```python
from build123d import *

# Parameters (mm, degrees)
CYLINDER950_R          = 0.9
CYLINDER950_DEPTH      = 15
CYLINDER950_ROLL_ANGLE = 90
CYLINDER951_R          = 0.9
CYLINDER951_DEPTH      = 15
CYLINDER951_ROLL_ANGLE = 90
BOX558_W               = 5
BOX558_H               = 60
BOX558_DEPTH           = 17
BOX557_W               = 7
BOX557_H               = 15
BOX557_DEPTH           = 17
FILLET357_R            = 3


with BuildPart() as cylinder1101:
    # Cylinder950 → Cylinder950 (new body)
    with BuildSketch(Plane.XY):
        Circle(CYLINDER950_R)
    extrude(amount=CYLINDER950_DEPTH)


with BuildPart() as cylinder1101_1:
    # Cylinder950 roll: moved
    add(cylinder1101.part.rotate(Axis((0, 0, 0), (1, 0, 0)), CYLINDER950_ROLL_ANGLE))


with BuildPart() as cylinder1101_2:
    # Cylinder950 placement: moved
    add(cylinder1101_1.part.moved(Location((27, 85, -10.2))))


with BuildPart() as fusion596:
    # Cylinder951 → Cylinder951 (new body)
    with BuildSketch(Plane.XY):
        Circle(CYLINDER951_R)
    extrude(amount=CYLINDER951_DEPTH)


with BuildPart() as fusion596_1:
    # Cylinder951 roll: moved
    add(fusion596.part.rotate(Axis((0, 0, 0), (1, 0, 0)), CYLINDER951_ROLL_ANGLE))


with BuildPart() as fusion596_2:
    # Cylinder951 placement: moved
    add(fusion596_1.part.moved(Location((27, 85, 0))))

    # Fusion596: union Cylinder1101
    add(cylinder1101_2.part)


with BuildPart() as fusion596_3:
    # Fusion596 placement: moved
    add(fusion596_2.part.moved(Location((44.2, 9.5, -5.9))))


with BuildPart() as cube749:
    # Box558 → Box558 (new body)
    with BuildSketch(Plane(origin=(74.5, 55, -19.5), x_dir=(1, 0, 0), z_dir=(0, 0, 1))):
        with Locations((2.5, 30)):
            Rectangle(BOX558_W, BOX558_H)
    extrude(amount=BOX558_DEPTH)


with BuildPart() as steering_servo_rear_mount:
    # Box557 → Box557 (new body)
    with BuildSketch(Plane(origin=(67.5, 79.5, -19.5), x_dir=(1, 0, 0), z_dir=(0, 0, 1))):
        with Locations((3.5, 7.5)):
            Rectangle(BOX557_W, BOX557_H)
    extrude(amount=BOX557_DEPTH)

    # Fusion597: union Cube749
    add(cube749.part)

    # Cut695: cut Fusion596
    add(fusion596_3.part, mode=Mode.SUBTRACT)

    # Fillet357
    fillet357_edges = [steering_servo_rear_mount.edges().sort_by_distance(p)[0] for p in [
        (77, 55, -2.5),
        (77, 115, -2.5),
        (77, 115, -19.5),
        (77, 55, -19.5),
    ]]
    fillet(fillet357_edges, radius=FILLET357_R)


with BuildPart() as steering_servo_rear_mount_1:
    # Fillet357 placement: moved
    add(steering_servo_rear_mount.part.moved(Location((1, 0, 0))))


solid = steering_servo_rear_mount_1.part
```
CAD build for the part. Positions are in the model's coordinates, mm. A direction names the side the tool comes from. Coordinates: 2 decimals unless noted, no trailing zeros. Order: outer loops, then holes, each group sorted by start corner. A loop starts at its lowest first (then second) coordinate and runs counter-clockwise, first axis right, second up. Notation, with made-up numbers: M 10.25,46.5 L 19.25,46.5 A14 cw 19.25,69.5 Z; hole C 31,52.25 d7. An arc over 180 degrees is marked long. Answer as CSV lines item,"result".
1) Mould opens along Z. For faces 1 (the flat face through (77, 85, -2.5)), 2 (the flat face through (80.5, 85, -11)), 3 (the cylindrical face through (71.3, 87.1, -5.9)), 4 (the cylindrical face through (71.3, 87.1, -16.1)) say: released by +Z, released by -Z, zero draft, split by the parting line, or undercut.
Verdict:
face 1,"released by +Z"
face 2,"zero draft"
face 3,"undercut"
face 4,"undercut"
2) Cut at B-B (z = -10.5). List the corners of the cut face in (x, y).
Verdict:
outline,"M 68.5,79.5 L 75.5,79.5 L 75.5,55 L 80.5,55 L 80.5,115 L 75.5,115 L 75.5,94.5 L 68.5,94.5 Z"
3) Cut at A-A (x = 72.2). List the corners of the cut face in (y, z).
Verdict:
outline,"M 79.5,-19.5 L 94.5,-19.5 L 94.5,-17 L 79.5,-17 Z; M 79.5,-15.2 L 94.5,-15.2 L 94.5,-6.8 L 79.5,-6.8 Z; M 79.5,-5 L 94.5,-5 L 94.5,-2.5 L 79.5,-2.5 Z"
4) Drill centre lines: L1, parallel to Z at x = 72.2, y = 83; L2, parallel to X at y = 89, z = -16.1; L3, parallel to Y at x = 72.5, z = -18.5. Where is each one in solid material? Low to high. Write a range as from..to.
Verdict:
L1,"-19.5..-17, -15.2..-6.8, -5..-2.5"
L2,"68.5..71.3, 73.1..80.5"
L3,"79.5..94.5"
5) Cut at C-C (y = 88.5). List the corners of the cut face in (x, z).
Verdict:
outline,"M 68.5,-19.5 L 80.5,-19.5 L 80.5,-2.5 L 68.5,-2.5 Z; hole C 72.2,-16.1 d1.8; hole C 72.2,-5.9 d1.8"
6) 3-axis set-ups, long thin cutter, end or side, ignore diameter. For faces 5 (the cylindrical face through (78.04, 55.9, -3.36)), 6 (the flat face through (72, 94.5, -11)), 7 (the flat face through (75.5, 67, -11)): which of +Z, -Z, +X, -X, +Y, -Y reach the whole face in a straight line?
Verdict:
face 5,"+Z, +X, -X, -Y"
face 6,"+Z, -Z, -X, +Y"
face 7,"+Z, -Z, -X, -Y"
7) Flat gauge pins, fed straight in: P1, Ø2, axis at y = 64.5, z = -6, coming from the -X side; P2, Ø3.5, axis at x = 70.5, z = -11.5, coming from the +Y side; P3, Ø1.4, axis at x = 72.2, z = -5.9, coming from the +Y side; P4, Ø2, axis at x = 72, z = -12, coming from the -Y side. Where does each tip first touch, or does it go through?
Verdict:
P1,"x = 75.5"
P2,"y = 94.5"
P3,"through"
P4,"y = 79.5"
8) Cut at D-D (x = 74.75). List the corners of the cut face in (y, z), then the cut area to 3 significant figures.
Verdict:
outline,"M 79.5,-19.5 L 94.5,-19.5 L 94.5,-2.5 L 79.5,-2.5 Z"
area,"255 mm2"
